Geometry: final body of the model. Coordinates: model frame, mm. A direction names the side the tool comes from. Give positions to 0.01 mm unless a question says otherwise; leave off trailing zeros. Loops run counter-clockwise (first coordinate to the right, second up) from the corner with the lowest first, then second, coordinate; pieces in that order, holes last.
1. Material intervals for line 1 along Z through (x, y) = (-2.25, -4.5); line 2 along Y through (x, z) = (5.5, 21.75); line 3 along Z through (x, y) = (-2.5, 0.5), sorted ascending.
2. Section A-A, the plane y = 0. Output: boundary loops of the cut face in (x, z), then the cut area to 3 significant figures.
3. Section B-B, the plane z = 16.25. Output: boundary loops of the cut face in (x, y).
4. Access query for faces 1 (the face through (0, 0, 0)), 2 (the face through (-1.5, 2.6, 22)), 3 (the face through (-0.867, 3.905, 8.294)). Directions: +Z, -Z, +X, -X, +Y, -Y. A direction counts if a zero-diameter tool reaches every point of the face in a straight line with its end or side. Return the directions, or none.
5. First-contact query: P1, Ø5, axis at x = -3, y = 5, coming from the -Z side; P2, Ø1, axis at x = 2, y = -5, coming from the -Z side; P3, Ø3, axis at x = -0.5, z = 7.5, coming from the +Y side. Flat tips, straight axial feed; report the tip coordinate or a pass-through.
6. Section C-C, the plane z = 11.75. Output: boundary loops of the cut face in (x, y), then the cut area to 3 significant figures.
Autodesk Inventor part; units mm, degrees
ref_plane "YZ Plane" through (0, 0, 0) normal (1, 0, 0) x (0, 1, 0)
ref_plane "XZ Plane" through (0, 0, 0) normal (0, 1, 0) x (-1, 0, 0)
ref_plane "XY Plane" through (0, 0, 0) normal (0, 0, 1) x (1, 0, 0)
sketch "Sketch1" plane through (0, 0, 0) normal (0, 0, 1) x (1, 0, 0)
  circle A0 centre (0, 0) radius 4
  dimension "Diameter" = 8
extrude "Extrusion1" add sketch "Sketch1" along normal blind 16
sketch "Sketch2" plane through (0, 0, 16) normal (0, 0, 1) x (1, 0, 0)
  circle A0 centre (0, 0) radius 4
  circle A1 centre (0, 0) radius 6.5
  dimension "Head_Diameter" = 13
extrude "Extrusion2" add sketch "Sketch2" along normal blind 8 contours A0 | A1
sketch "Sketch3" plane through (0, 0, 24) normal (0, 0, 1) x (1, 0, 0)
  circle A0 centre (0, 0) radius 6.5
  circle A1 centre (0, 0) radius 3.4641 construction
  line L0 (0, 3.4641) -> (3, 1.7321)
  line L1 (3, -1.7321) -> (3, 1.7321)
  line L2 (0, 3.4641) -> (-3, 1.7321)
  line L3 (-3, -1.7321) -> (-3, 1.7321)
  line L4 (-3, -1.7321) -> (0, -3.4641)
  line L5 (3, -1.7321) -> (0, -3.4641)
  dimension "Hex_Width" = 6
extrude "Extrusion3" cut sketch "Sketch3" against normal blind 4 contours L0 L1 L5 L4 L3 L2
thread "Thread1"
chamfer "Chamfer1" distance 0.8 angle 45 2 edges at (-6.5, 0, 24) (-4, 0, 0)
equation "\"d9\" = ThreadLength"
equation "\"d12\" = Chamfer"
equation "\"ThreadLength\" = 16"
properties part number "SCREW,SOCKET HD,P,12.9,M8X1.25X16MM"
Answers below:
1. line 1: z = 16 to 24
1. line 2: y = -3.46 to 3.46
1. line 3: z = 0 to 20
2. outline: (-6.5, 16) - (-4, 16) - (-4, 0.8) - (-3.2, 0) - (3.2, 0) - (4, 0.8) - (4, 16) - (6.5, 16) - (6.5, 23.2) - (5.7, 24) - (3, 24) - (3, 20) - (-3, 20) - (-3, 24) - (-5.7, 24) - (-6.5, 23.2) - close
2. area: 207 mm2
3. outline: circle Ø13 at (0, 0)
4. face 1: -Z, +X, -X, +Y, -Y
4. face 2: +Z
4. face 3: -Z
5. P1: stops at z = 0.13
5. P2: stops at z = 16
5. P3: stops at y = 4
6. outline: circle Ø8 at (0, 0)
6. area: 50.3 mm2
